```python
from build123d import *

# Parameters (mm, degrees)
SKETCH_1_R      = 10.65
SKETCH_1_R_2    = 8.65
EXTRUDE_1_DEPTH = 64.5


with BuildPart() as part:
    # Эскиз1 → Бобышка-Вытянуть1 (new body)
    with BuildSketch(Plane(origin=(0, 0, 0), x_dir=(0, 0, -1), z_dir=(1, 0, 0))):
        Circle(SKETCH_1_R)
        Circle(SKETCH_1_R_2, mode=Mode.SUBTRACT)
    extrude(amount=-EXTRUDE_1_DEPTH)

    # Эскиз2 → Вырез-Повернуть1 (revolve, cut)
    with BuildSketch(Plane.XY):
        Polygon((-38.480196097, 10.65), (-64.5, 10.65), (-64.5, 10), (-50.980196097, 10), (-50.980196097, 10.4), (-38.480196097, 10.4), align=None)
    revolve(axis=Axis((-1000, 0, 0), (1, 0, 0)), mode=Mode.SUBTRACT)

    # Зеркальное отражение1: part across plane


with BuildPart() as part_1:
    add(part.part)
    add(part.part.mirror(Plane(origin=(0, 0, 0), x_dir=(0, 0, 1), z_dir=(1, 0, 0))))


solid = part_1.part
```
The listing builds one solid part. Answer for the finished solid, in the listing's coordinates (mm). A direction names the side the tool comes from. Give positions to 0.01 mm unless a question says otherwise; leave off trailing zeros. Order: outer loops, then holes, each group sorted by start corner. A loop starts at its lowest first (then second) coordinate and runs counter-clockwise, first axis right, second up.
1) Given P1, Ø8, axis at x = 22, y = -7.5, coming from the +Z side; P2, Ø1.5, axis at x = 16.5, z = -1.5, coming from the -Y side; P3, Ø5, axis at x = 16, z = 5.5, coming from the +Y side; P4, Ø10.5, axis at y = 0.5, z = 2.5, coming from the -X side, each flat-ended and moving along its own axis, determine where each tip first touches the part or whether it passes through.
Reported:
P1: stops at z = 10.06
P2: stops at y = -10.62
P3: stops at y = 10.22
P4: passes through
2) Find section D-D on x = 2. Write down the section's boundary in (y, z), then the cut area to 3 significant figures.
Reported:
outline: circle Ø21.3 at (0, 0); hole circle Ø17.3 at (0, 0)
area: 121 mm2
3) Find section A-A on y = 0. Write down the section's boundary in (x, z), then the cut area to 3 significant figures.
Reported:
outline: (-64.5, -10) - (-50.98, -10) - (-50.98, -10.4) - (-38.48, -10.4) - (-38.48, -10.65) - (38.48, -10.65) - (38.48, -10.4) - (50.98, -10.4) - (50.98, -10) - (64.5, -10) - (64.5, -8.65) - (-64.5, -8.65) - close; (-64.5, 8.65) - (64.5, 8.65) - (64.5, 10) - (50.98, 10) - (50.98, 10.4) - (38.48, 10.4) - (38.48, 10.65) - (-38.48, 10.65) - (-38.48, 10.4) - (-50.98, 10.4) - (-50.98, 10) - (-64.5, 10) - close
area: 468 mm2
4) For faces 1 (the face through (-57.65, -2.17, -9.76)), 2 (the face through (64.5, 7, 6)), 3 (the face through (44.64, -1.35, 10.31)), determine the directions among +Z, -Z, +X, -X, +Y, -Y from which every point of the face is accessible in a straight line to the end or side of a thin tool.
Reported:
face 1: -X
face 2: +Z, -Z, +X, +Y, -Y
face 3: +X
5) Find section C-C on x = 41.5. Write down the section's boundary in (y, z), then the cut area to 3 significant figures.
Reported:
outline: circle Ø20.8 at (0, 0); hole circle Ø17.3 at (0, 0)
area: 105 mm2
6) Consider line 1 along Y through (x, z) = (3.5, 0.5); line 2 along Z through (x, y) = (11.5, 6.75); line 3 along Z through (x, y) = (23.5, -2.5). Determine where each line is inside the solid, lowest interval first.
Reported:
line 1: y = -10.64 to -8.64, 8.64 to 10.64
line 2: z = -8.24 to -5.41, 5.41 to 8.24
line 3: z = -10.35 to -8.28, 8.28 to 10.35
